Geometry check sheet. Reference: the model listing, model coordinates, mm. Coordinates: 2 decimals unless noted, no trailing zeros. Write each loop counter-clockwise with the first axis right and the second up, starting at its lowest first coordinate (ties: lowest second). Pieces come first, ordered by that corner, then holes. Notation, with made-up numbers: M -36.5,54 L -17.5,54 A23 cw -17.5,93 Z; hole C -7,82 d5. An arc over 180 degrees is marked long. Put each result on its own line as item: value. Start each with the question number.
1) Cross-section at A-A on x = 897. Record the cut outline in (y, z).
2) Scan lines: line 1 along Z through (x, y) = (1097, 50); line 2 along X through (y, z) = (38.5, 49.5); line 3 along X through (y, z) = (7.5, 7). Record each from-to range of solid material in increasing order.
3) Gauge pin test, flat ends, axial feed: pin 1 (10.5 mm diameter, centred on y = 50.5, z = 9, fed in from +X); pin 2 (11.5 mm diameter, centred on x = -331.79, z = -8.73, fed in from -Y); pin 3 (6.5 mm diameter, centred on x = 1010, z = 7.5, fed in from -Y). Record the tip position at first contact, or that the pin passes through.
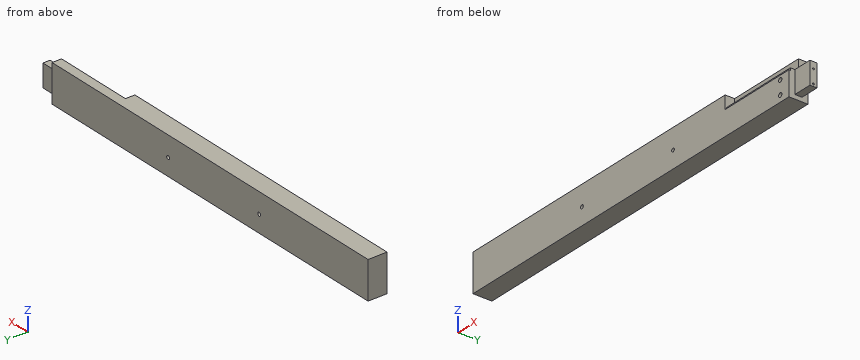
from build123d import *

# Parameters (mm, degrees)
SKETCH1_W           = 2136.775
SKETCH1_H           = 201.6125
BOSS_EXTRUDE1_DEPTH = 101.6
SKETCH2_R           = 9.525
CUT_EXTRUDE1_DEPTH  = 1078.931496059
SKETCH3_W           = 120.65
SKETCH3_H           = 38.1
SKETCH3_R           = 4.7625
BOSS_EXTRUDE2_DEPTH = 101.6
CUT_EXTRUDE2_DEPTH  = 431.8
SKETCH5_R           = 11.1125
CUT_EXTRUDE3_DEPTH  = 69.85


with BuildPart() as part:
    # Sketch1 → Boss-Extrude1 (new body)
    with BuildSketch(Plane(origin=(0, 0, 0), x_dir=(1, 0, 0), z_dir=(0, 1, 0))):
        Rectangle(SKETCH1_W, SKETCH1_H)
    extrude(amount=BOSS_EXTRUDE1_DEPTH)

    # Sketch2 → Cut-Extrude1 (cut, through all)
    with BuildSketch(Plane(origin=(0, 101.6, 0), x_dir=(1, 0, 0), z_dir=(0, 1, 0))):
        with Locations(Location((-331.7875, 8.73125, 0), (0, 0, 270))):
            Circle(SKETCH2_R)
        with Locations(Location((284.1625, 8.73125, 0), (0, 0, 270))):
            Circle(SKETCH2_R)
    extrude(amount=-CUT_EXTRUDE1_DEPTH, mode=Mode.SUBTRACT)

    # Sketch3 → Boss-Extrude2 (add)
    with BuildSketch(Plane(origin=(1068.3875, 0, 0), x_dir=(0, 0, -1), z_dir=(1, 0, 0))):
        with Locations((18.25625, 50.8)):
            Rectangle(SKETCH3_W, SKETCH3_H)
        with Locations((-7.14375, 50.8)):
            Circle(SKETCH3_R, mode=Mode.SUBTRACT)
        with Locations((65.88125, 50.8)):
            Circle(SKETCH3_R, mode=Mode.SUBTRACT)
    extrude(amount=BOSS_EXTRUDE2_DEPTH)

    # Sketch3_3 → Cut-Extrude2 (cut)
    with BuildSketch(Plane(origin=(1068.3875, 0, 0), x_dir=(0, 0, -1), z_dir=(1, 0, 0))):
        Polygon((-42.06875, 31.75), (-42.06875, 50.8), (-100.80625, 50.8), (-100.80625, 0), (-29.932015023, 0), (-29.932015023, 7.312255735), (-42.06875, 7.312255735), align=None)
    extrude(amount=-CUT_EXTRUDE2_DEPTH, mode=Mode.SUBTRACT)

    # Sketch5 → Cut-Extrude3 (cut)
    with BuildSketch(Plane.XZ):
        with Locations(Location((1009.306684953, 7.14375, 0), (0, 0, 270))):
            Circle(SKETCH5_R)
        with Locations(Location((1009.306684953, -65.88125, 0), (0, 0, 270))):
            Circle(SKETCH5_R)
    extrude(amount=-CUT_EXTRUDE3_DEPTH, mode=Mode.SUBTRACT)


solid = part.part
Answer key:
1. outline: M 0,-100.81 L 101.6,-100.81 L 101.6,100.81 L 50.8,100.81 L 50.8,42.07 L 7.31,42.07 L 7.31,29.93 L 0,29.93 Z
2. line 1: z = -78.58 to -70.58, -61.19 to 2.45, 11.84 to 42.07
2. line 2: x = -1068.39 to 636.59
2. line 3: x = -1068.39 to 998.2, 1020.42 to 1068.39
3. pin 1: stops at x = 1169.99
3. pin 2: passes through
3. pin 3: stops at y = 69.85
